Autodesk Inventor part; units mm, degrees
ref_plane "YZ Plane" through (0, 0, 0) normal (1, 0, 0) x (0, 1, 0)
ref_plane "XZ Plane" through (0, 0, 0) normal (0, 1, 0) x (-1, 0, 0)
ref_plane "XY Plane" through (0, 0, 0) normal (0, 0, 1) x (1, 0, 0)
sketch "Sketch1" plane through (0, 0, 0) normal (0, 0, 1) x (1, 0, 0)
  arc A0 (0, -7.5) -> (0, 7.5) centre (0, 0) ccw
  line L0 (0, -7.5) -> (0, 7.5)
  dimension "d5" = 15
revolve "Revolution1" add sketch "Sketch1" angle 360 about axis through (0, -7.5, 0) along (0, 1, 0)
sketch "Sketch2" plane through (0, 0, 0) normal (0, 0, 1) x (1, 0, 0)
  circle A0 centre (0, 0) radius 6
  dimension "d2" = 12
extrude "Extrusion1" add sketch "Sketch2" along normal blind 7
sketch "Sketch3" plane through (0, 0, 7) normal (0, 0, 1) x (1, 0, 0)
  circle A0 centre (0, 0) radius 6
  line L0 (-4.0415, 7) -> (4.0415, 7)
  line L1 (4.0415, 7) -> (8.0829, 0)
  line L2 (8.0829, 0) -> (4.0415, -7)
  line L3 (4.0415, -7) -> (-4.0415, -7)
  line L4 (-4.0415, -7) -> (-8.0829, 0)
  line L5 (-8.0829, 0) -> (-4.0415, 7)
  point P0 (0, -7)
  dimension "d6" = 120
  dimension "d7" = 120
  dimension "d8" = 14
extrude "Extrusion2" add sketch "Sketch3" along normal blind 7.5 contours A0 | L0 L1 L2 L3 L4 L5
sketch "Sketch4" plane through (0, 0, 14.5) normal (0, 0, 1) x (1, 0, 0)
  circle A0 centre (0, 0) radius 5
  point P0 (0, 0)
  dimension "d11" = 10
extrude "Extrusion3" add sketch "Sketch4" along normal blind 90
thread "Thread1"
chamfer "Chamfer1" distance 1 angle 45 1 edges at (-5, 0, 104.5)
properties part number "21.1846 THREADED STUD 10mm" material "Steel"
Can you work these out from the model? Positions are in its coordinate system, mm. A direction names the side the tool comes from. Round coordinates to 2 decimals unless told otherwise and drop trailing zeros. Order: outer loops, then holes, each group sorted by start corner. A loop starts at its lowest first (then second) coordinate and runs counter-clockwise, first axis right, second up. Notation, with made-up numbers: (60.5, 35.25) - (86.5, 35.25) arc R16 cw to (86.5, 39.25) - close; hole circle Ø4 at (73.25, -37.5). An arc over 180 degrees is marked (long way). Answer in a Markdown table with one row per item.
(1) Please list where these lines run through material, in increasing order: L1, parallel to X at y = -0.25, z = 59.5; L2, parallel to Y at x = -2.75, z = 10.5; L3, parallel to Z at x = -5.75, y = -2.75. Write a range as from..to.
From the geometry:
| item | result |
|---|---|
| L1 | x = -4.99..4.99 |
| L2 | y = -7..7 |
| L3 | z = -3.95..3.95, 7..14.5 |
(2) If we mould it in two halves opening along Z, with no side actions, what happens to faces 6 (the face through (0, 0, 104.5)), 7 (the face through (-6.09, 3.45, 10.7)), 8 (the face through (-2, 6, 7))? For each: released by +Z, released by -Z, zero draft, split by the parting line, or undercut.
From the geometry:
| item | result |
|---|---|
| face 6 | released by +Z |
| face 7 | zero draft |
| face 8 | undercut |
(3) Suppose I cut it at A-A, the plane z = 11. Please give me the cut outline in (x, y).
From the geometry:
| item | result |
|---|---|
| outline | (-8.08, 0) - (-4.04, -7) - (4.04, -7) - (8.08, 0) - (4.04, 7) - (-4.04, 7) - close |
(4) Which directions (+Z, -Z, +X, -X, +Y, -Y) give clear straight access to the entire face, cutting with the end or side of a thin tool? Please do faces 1 (the face through (0, 7, 11)), 2 (the face through (0, -7, 11)), 3 (the face through (6.034, 3.549, 10.698)), 4 (the face through (-6.034, -3.549, 10.698)), 5 (the face through (-1.08, 4.88, 58.38)).
From the geometry:
| item | result |
|---|---|
| face 1 | +Z, +X, -X, +Y |
| face 2 | +Z, +X, -X, -Y |
| face 3 | +Z, +X, +Y |
| face 4 | +Z, -X, -Y |
| face 5 | +Z |
(5) Suppose I cut it at C-C, the plane z = 55. Please give me the cut outline in (x, y), plus the area to 3 significant figures.
From the geometry:
| item | result |
|---|---|
| outline | circle Ø10 at (0, 0) |
| area | 78.5 mm2 |
(6) Suppose I cut it at B-B, the plane x = 0. Please give me the cut outline in (y, z), plus the area to 3 significant figures.
From the geometry:
| item | result |
|---|---|
| outline | (-7, 7) - (-6, 7) - (-6, 4.5) arc R7.5 ccw (long way) to (6, 4.5) - (6, 7) - (7, 7) - (7, 14.5) - (5, 14.5) - (5, 103.5) - (4, 104.5) - (-4, 104.5) - (-5, 103.5) - (-5, 14.5) - (-7, 14.5) - close |
| area | 1,190 mm2 |
(7) For P1, Ø1, axis at x = -5.5, y = 3, coming from the -Z side; P2, Ø8, axis at x = -5, y = -1, coming from the -Z side; P3, Ø2, axis at x = -0.5, z = 12, coming from the +Y side, each with a flat end and sliding along its axis, tell me the tip position at first contact or that it passes through.
From the geometry:
| item | result |
|---|---|
| P1 | stops at z = -4.8 |
| P2 | stops at z = -7.42 |
| P3 | stops at y = 7 |
